The listing builds one solid part. Answer for the finished solid, in the listing's coordinates (mm). A direction names the side the tool comes from. Coordinates: 2 decimals unless noted, no trailing zeros. Order: outer loops, then holes, each group sorted by start corner. A loop starts at its lowest first (then second) coordinate and runs counter-clockwise, first axis right, second up.
```python
from build123d import *

# Parameters (mm, degrees)
F1_DEPTH  = 4.5
F3_DEPTH  = 6
F5_DEPTH  = 4.5
F6_R      = 9
F7_DEPTH  = 4.5
F8_R      = 9
F9_DEPTH  = 4.5
F11_DEPTH = 10.501
F12_R     = 1.5
F13_DEPTH = 15.001
F14_R     = 2.5
F15_DEPTH = 1.5
F16_R     = 2.5
F17_DEPTH = 1.5
F18_R     = 48.9418090598
F19_DEPTH = 12.5


with BuildPart() as f1:
    # F0 (on Right) → F1 (new body)
    with BuildSketch(Plane.YZ):
        with BuildLine():
            ThreePointArc((24.9939795279, 8.4831504125), (13.3131715809, 6.0580646826), (1.4100295584, 6.8565163636))
            ThreePointArc((1.4100295584, 6.8565163636), (-7, 0), (1.4100295584, -6.8565163636))
            ThreePointArc((1.4100295584, -6.8565163636), (13.3131715809, -6.0580646826), (24.9939795279, -8.4831504125))
            ThreePointArc((24.9939795279, -8.4831504125), (37, 0), (24.9939795279, 8.4831504125))
        make_face()
    extrude(amount=F1_DEPTH)

    # F2 (on face) → F3 (join)
    with BuildSketch(Plane.YZ.offset(4.5)):
        with BuildLine():
            ThreePointArc((24.9939795279, 8.4831504125), (13.3131715809, 6.0580646826), (1.4100295584, 6.8565163636))
            ThreePointArc((1.4100295584, 6.8565163636), (0.7086555774, 6.9640367082), (0, 7))
            Line((0, 7), (0, 5.5))
            ThreePointArc((0, 5.5), (2.9705148408, 4.628827236), (5, 2.2912878475))
            Line((5, 2.2912878475), (8.7899052004, -5.9789633228))
            ThreePointArc((8.7899052004, -5.9789633228), (17.0094937021, -6.4704065852), (24.9939795279, -8.4831504125))
            ThreePointArc((24.9939795279, -8.4831504125), (37, 0), (24.9939795279, 8.4831504125))
        make_face()
    extrude(amount=F3_DEPTH)

    # F4 (on face) → F5 (join)
    with BuildSketch(Plane.YZ.offset(10.5)):
        with BuildLine():
            ThreePointArc((1.4100295584, 6.8565163636), (0.7086555774, 6.9640367082), (0, 7))
            ThreePointArc((0, 7), (-6.9640367082, -0.7086555774), (1.4100295584, -6.8565163636))
            ThreePointArc((1.4100295584, -6.8565163636), (5.0814258107, -6.261812549), (8.7899052004, -5.9789633228))
            ThreePointArc((8.7899052004, -5.9789633228), (17.0094937021, -6.4704065852), (24.9939795279, -8.4831504125))
            ThreePointArc((24.9939795279, -8.4831504125), (26.6900035871, -8.9041512452), (28.4354151468, -8.9894612547))
            ThreePointArc((28.4354151468, -8.9894612547), (36.8303478161, 1.7392404799), (24.9939795279, 8.4831504125))
            ThreePointArc((24.9939795279, 8.4831504125), (13.3131715809, 6.0580646826), (1.4100295584, 6.8565163636))
        make_face()
    extrude(amount=F5_DEPTH)

    # F6 (on face) → F7 (cut)
    with BuildSketch(Plane.YZ.offset(15)):
        with Locations((28, 0)):
            Circle(F6_R)
    extrude(amount=-F7_DEPTH, mode=Mode.SUBTRACT)

    # F8 (on face) → F9 (cut)
    with BuildSketch(Plane(origin=(0, 0, 0), x_dir=(0, -1, 0), z_dir=(-1, 0, 0))):
        with Locations((-28, 0)):
            Circle(F8_R)
    extrude(amount=-F9_DEPTH, mode=Mode.SUBTRACT)

    # F10 (on face) → F11 (cut, through all)
    with BuildSketch(Plane.YZ.offset(10.5)):
        with BuildLine():
            ThreePointArc((28, 7), (34.6787700412, 2.0961943462), (32, -5.7445626465))
            Line((32, -5.7445626465), (27.3576923402, -8.9770507891))
            ThreePointArc((27.3576923402, -8.9770507891), (36.9942608674, -0.3213587544), (28, 9))
            Line((28, 9), (28, 7))
        make_face()
    extrude(amount=-F11_DEPTH, mode=Mode.SUBTRACT)

    # F12 (on face) → F13 (cut, through all)
    with BuildSketch(Plane.YZ.offset(15)):
        Circle(F12_R)
        with Locations((28, 0)):
            Circle(F12_R)
    extrude(amount=-F13_DEPTH, mode=Mode.SUBTRACT)

    # F14 (on face) → F15 (cut)
    with BuildSketch(Plane.YZ.offset(15)):
        Circle(F14_R)
    extrude(amount=-F15_DEPTH, mode=Mode.SUBTRACT)

    # F16 (on face) → F17 (cut)
    with BuildSketch(Plane(origin=(0, 0, 0), x_dir=(0, -1, 0), z_dir=(-1, 0, 0))):
        Circle(F16_R)
    extrude(amount=-F17_DEPTH, mode=Mode.SUBTRACT)

    # F18 (on Top) → F19 (cut, symmetric)
    with BuildSketch(Plane.XY):
        with Locations((-47.5, 13.2020045432)):
            Circle(F18_R)
        with Locations((62.5, 13.2020045432)):
            Circle(F18_R)
    extrude(amount=F19_DEPTH, both=True, mode=Mode.SUBTRACT)


solid = f1.part
```
(1) Consider line 1 (X direction, y = -2, z = -2.75); line 2 (Z direction, x = 3.5, y = 0); line 3 (X direction, y = 25.5, z = -3). Determine where each line is inside the solid, lowest interval first.
(2) For faces 5 (the face through (1.5, 0, -2)), 6 (the face through (7, 0, 6)), 7 (the face through (8, 28, 8)), 8 (the face through (12, 19, 0)), determine the directions among +Z, -Z, +X, -X, +Y, -Y from which every point of the face is accessible in a straight line to the end or side of a thin tool.
(3) Find section A-A (x = 6). Write down the section's boundary in (y, z).
(4) The mould has two halves that part along Z. Classify faces 1 (the face through (7.4, 13.48, 6.07)), 2 (the face through (4.5, 0.8, -1.5)), 3 (the face through (7.458, 2.933, 4.652)), 4 (the face through (14.3, -2.5, 0.1)): released by +Z, released by -Z, zero draft, split by the parting line, or undercut.
(5) Each of these flat-tipped pins is pushed along its axis until it touches: pin 1 Ø1 at (x, z) = (8, -2) entering from -Y; pin 2 Ø4 at (y, z) = (0, 0) entering from +X; pin 3 Ø4 at (x, z) = (10, 3.5) entering from -Y; pin 4 Ø6 at (y, z) = (0, 0) entering from +X. Where does it stop, or does it pass through?
(6) Find section B-B (z = 0). Give the number of separate pieces and of enclosed holes in the cut face, and give its area (3 significant figures).
(7) Find section D-D (y = 21). Write down the section's boundary in (x, z), and give its area (3 significant figures).
(8) Find section C-C (z = 3.25). Write down the section's boundary in (x, y).
Findings below:
1. line 1: x = 0 to 4.5, 10.5 to 15
1. line 2: z = -7 to -1.5, 1.5 to 7
1. line 3: x = 4.5 to 10.5
2. face 5: -X
2. face 6: +Z, -Z, -Y
2. face 7: +Z, +X, -X, +Y
2. face 8: +X, +Y
3. outline: (0, 5.5) arc R5.5 cw to (5, 2.29) - (8.79, -5.98) arc R44.05 cw to (24.99, -8.48) arc R9 ccw to (27.36, -8.98) - (32, -5.74) arc R7 ccw to (28, 7) - (28, 9) arc R9 ccw to (24.99, 8.48) arc R44.05 cw to (1.41, 6.86) arc R7 ccw to (0, 7) - close; hole circle Ø3 at (28, 0)
4. face 1: released by +Z
4. face 2: zero draft
4. face 3: released by -Z
4. face 4: undercut
5. pin 1: stops at y = 6.74
5. pin 2: stops at x = 13.5
5. pin 3: stops at y = -6.82
5. pin 4: stops at x = 15
6. separate pieces: 4
6. enclosed holes: 0
6. area: 319 mm2
7. outline: (0.82, -7.28) - (14.18, -7.28) - (14.18, -5.66) - (10.5, -5.66) - (10.5, 5.66) - (14.18, 5.66) - (14.18, 7.28) - (0.82, 7.28) - (0.82, 5.66) - (4.5, 5.66) - (4.5, -5.66) - (0.82, -5.66) - close
7. area: 111 mm2
8. outline: (0, -6.2) - (4.5, -6.2) - (4.5, 4.44) - (10.5, 4.44) - (10.5, -6.2) - (15, -6.2) - (15, 1.41) arc R48.94 cw to (13.98, 19.61) - (10.5, 19.61) - (10.5, 34.2) - (4.5, 34.2) - (4.5, 19.61) - (1.02, 19.61) arc R48.94 cw to (0, 1.41) - close
